Work out the finished part from the listing and answer in its coordinate system (mm). A direction names the side the tool comes from. Coordinates: 2 decimals unless noted, no trailing zeros. Write each loop counter-clockwise with the first axis right and the second up, starting at its lowest first coordinate (ties: lowest second). Pieces come first, ordered by that corner, then holes. Notation, with made-up numbers: (43, 86) - (57, 86) arc R19 ccw to (57, 112) - close; hole circle Ø3 at (60.5, 28). An arc over 180 degrees is marked (long way). Use a Markdown table: item, result. Add a question column.
(1) For a pull along Z with two mould halves and no side action, classify faces 1 (the face through (0.2, 10, 36.3)), 2 (the face through (-35.59, -0.14, -10.97)), 3 (the face through (36.16, -0.14, -13.16)) as released by +Z, released by -Z, zero draft, split by the parting line, or undercut.
(2) A tool of negligible diameter and unlimited length cuts with its end or side. For faces 4 (the face through (35.526, -0.14, -10.945)), 5 (the face through (-36.19, -0.14, -13.17)), from which of +Z, -Z, +X, -X, +Y, -Y can it reach the whole face along a straight path? Write none if from no direction.
(3) Find the intervals of material crossed by line 1 (X direction, y = 8, z = -3); line 2 (X direction, y = 7.25, z = 26); line 3 (Z direction, x = -20, y = 2.5), in increasing order. Write a range as from..to.
(4) Given pin 1 Ø10 at (y, z) = (-1.5, 9.5) entering from +X; pin 2 Ø10 at (y, z) = (-5.5, -1.5) entering from -X; pin 3 Ø10 at (x, y) = (13.5, -5) entering from -Z, each flat-ended and moving along its own axis, determine where each tip first touches the part or whether it passes through.
(5) The part is cut by section A-A, the plane y = -0.75. Give the vertices of the cut face in (x, z).
from build123d import *

# Parameters (mm, degrees)
FUNDAMETAL_DIMENSIONS_DEPTH           = 10
FUNDAMETAL_DIMENSIONS_DEPTH_BACK      = 10
ROUND_INSIDE_CUT_ANGLE                = 110
ROUND_INSIDE_CUT_OTHER_WAY_ANGLE      = 110
ROUND_INSIDE_EXTRUDED_ANGLE           = 110
ROUND_INSIDE_EXTRUDED_OTHER_WAY_ANGLE = 110


with BuildPart() as part:
    # Sketch3 → Fundametal Dimensions (new, two sides: drawn at the far end of the back side and taken through both)
    with BuildSketch(Plane(origin=(0, 0, 0), x_dir=(1, 0, 0), z_dir=(0, 1, 0)).offset(-FUNDAMETAL_DIMENSIONS_DEPTH_BACK)):
        with BuildLine():
            Line((-36.955795179, 13.450809429), (-35.392364764, 12.881767294))
            ThreePointArc((-35.392364764, 12.881767294), (-35.560736729, 10.95726692), (-34.452672143, 12.539747151))
            Line((-34.452672143, 12.539747151), (-32.889241728, 11.970705016))
            ThreePointArc((-32.889241728, 11.970705016), (0, -35), (32.889241728, 11.970705016))
            Line((32.889241728, 11.970705016), (34.452672143, 12.539747151))
            ThreePointArc((34.452672143, 12.539747151), (35.560736729, 10.95726692), (35.392364764, 12.881767294))
            Line((35.392364764, 12.881767294), (36.955795179, 13.450809429))
            ThreePointArc((36.955795179, 13.450809429), (0, -39.327535793), (-36.955795179, 13.450809429))
        make_face()
    extrude(amount=FUNDAMETAL_DIMENSIONS_DEPTH + FUNDAMETAL_DIMENSIONS_DEPTH_BACK)

    # Sketch9 → Round Inside Cut (revolve, cut)
    with BuildSketch(Plane(origin=(0, 0, 0), x_dir=(0, 0, -1), z_dir=(1, 0, 0))):
        with BuildLine():
            Line((-36.099996489, 10), (-35, 10))
            Line((-35, 10), (-35, 5))
            ThreePointArc((-35, 5), (-35.45845478, 7.520139498), (-36.099996489, 10))
        make_face()
        with BuildLine():
            Line((-36.099996489, -10), (-35, -10))
            Line((-35, -10), (-35, -5))
            ThreePointArc((-35, -5), (-35.45845478, -7.520139498), (-36.099996489, -10))
        make_face()
    revolve(axis=Axis((0, -20, 0), (0, 1, 0)), revolution_arc=ROUND_INSIDE_CUT_ANGLE, mode=Mode.SUBTRACT)

    # Sketch9 → Round Inside Cut other way (revolve, cut)
    with BuildSketch(Plane(origin=(0, 0, 0), x_dir=(0, 0, -1), z_dir=(1, 0, 0))):
        with BuildLine():
            Line((-36.099996489, 10), (-35, 10))
            Line((-35, 10), (-35, 5))
            ThreePointArc((-35, 5), (-35.45845478, 7.520139498), (-36.099996489, 10))
        make_face()
        with BuildLine():
            Line((-36.099996489, -10), (-35, -10))
            Line((-35, -10), (-35, -5))
            ThreePointArc((-35, -5), (-35.45845478, -7.520139498), (-36.099996489, -10))
        make_face()
    revolve(axis=Axis((0, -20, 0), (0, -1, 0)), revolution_arc=ROUND_INSIDE_CUT_OTHER_WAY_ANGLE, mode=Mode.SUBTRACT)

    # Sketch10 → Round Inside Extruded (revolve)
    with BuildSketch(Plane(origin=(0, 0, 0), x_dir=(0, 0, -1), z_dir=(1, 0, 0))):
        with BuildLine():
            Line((-35, 5), (-35, -5))
            ThreePointArc((-35, -5), (-34.641016151, 0), (-35, 5))
        make_face()
    revolve(axis=Axis((0, -20, 0), (0, 1, 0)), revolution_arc=ROUND_INSIDE_EXTRUDED_ANGLE)

    # Sketch10 → Round Inside Extruded other way (revolve)
    with BuildSketch(Plane(origin=(0, 0, 0), x_dir=(0, 0, -1), z_dir=(1, 0, 0))):
        with BuildLine():
            Line((-35, 5), (-35, -5))
            ThreePointArc((-35, -5), (-34.641016151, 0), (-35, 5))
        make_face()
    revolve(axis=Axis((0, -20, 0), (0, -1, 0)), revolution_arc=ROUND_INSIDE_EXTRUDED_OTHER_WAY_ANGLE)


solid = part.part
Model answer:
| question | item | result |
|---|---|---|
| 1 | face 1 | zero draft |
| 1 | face 2 | undercut |
| 1 | face 3 | released by -Z |
| 2 | face 4 | +Y, -Y |
| 2 | face 5 | -Z, +Y, -Y |
| 3 | line 1 | -39.21..-35.44, 35.44..39.21 |
| 3 | line 2 | -29.51..-24.02, 24.02..29.51 |
| 3 | line 3 | 28.39..33.86 |
| 4 | pin 1 | x = 39.07 |
| 4 | pin 2 | x = -39.33 |
| 4 | pin 3 | z = 29.62 |
| 5 | outline | (-36.96, -13.45) - (-35.39, -12.88) arc R1 cw (long way) to (-34.45, -12.54) - (-32.56, -11.85) arc R34.65 cw (long way) to (32.56, -11.85) - (34.45, -12.54) arc R1 cw (long way) to (35.39, -12.88) - (36.96, -13.45) arc R39.33 ccw (long way) to start |
